Can you work these out from the model? Positions are in its coordinate system, mm. A direction names the side the tool comes from. Give positions to 0.01 mm unless a question says otherwise; leave off trailing zeros. Write each loop counter-clockwise with the first axis right and the second up, starting at its lowest first coordinate (ties: lowest second). Pieces come first, ordered by that corner, then holes. Notation, with made-up numbers: M -11,54.25 L 23,54.25 A18 cw 23,85.25 Z; hole C 19,31 d6. An arc over 180 degrees is marked long. Write each question's results on one line, items separated by ' | '.
from build123d import *

# Parameters (mm, degrees)
SKETCH2_R               = 3
CUT_EXTRUDE1_DEPTH      = 8.5
CUT_EXTRUDE1_DEPTH_BACK = 8.5
DOME1_FACE_RADIUS       = 6
DOME1_HEIGHT            = 2


with BuildPart() as part:
    # Sketch1 → Revolve1 (revolve)
    with BuildSketch(Plane.XY):
        Polygon((57, 0), (0, 0), (0, 6), (18, 6), (18, 5), (20, 5), (20, 7.5), (57, 7.5), align=None)
    revolve(axis=Axis((57, 0, 0), (-1, 0, 0)))

    # Sketch2 → Cut-Extrude1 (cut, two sides)
    with BuildSketch(Plane.XY) as cut_extrude1_sk:
        with Locations((48, 0)):
            Circle(SKETCH2_R)
    extrude(amount=CUT_EXTRUDE1_DEPTH, mode=Mode.SUBTRACT)
    extrude(cut_extrude1_sk.sketch, amount=-CUT_EXTRUDE1_DEPTH_BACK, mode=Mode.SUBTRACT)

    # Dome1: a dome of height H over a round flat face of radius A is a cap of a sphere of radius (A * A + H * H) / (2 * H)
    dome1_r = (DOME1_FACE_RADIUS * DOME1_FACE_RADIUS + DOME1_HEIGHT * DOME1_HEIGHT) / (2 * DOME1_HEIGHT)
    dome1_base = Plane((0, 0, 0), z_dir=(-1, 0, 0))
    with Locations(dome1_base.offset(DOME1_HEIGHT - dome1_r)):
        dome1_ball = Sphere(dome1_r, mode=Mode.PRIVATE)
    add(split(dome1_ball, bisect_by=dome1_base, keep=Keep.TOP, mode=Mode.PRIVATE))


solid = part.part
Item 1: I'm going to push flat-ended pins straight in: pin 1 (6 mm diameter, centred on x = 48.5, y = -3.5, fed in from +Z); pin 2 (1.5 mm diameter, centred on x = 50.5, y = -5, fed in from -Z); pin 3 (3 mm diameter, centred on x = 46, z = -4.5, fed in from +Y); pin 4 (5.5 mm diameter, centred on x = 48, y = 0, fed in from -Z). Where does each tip first touch, or does it pass through?
Geometry says:
pin 1: stops at z = 7.37 | pin 2: stops at z = -6.18 | pin 3: stops at y = 6.87 | pin 4: passes through
Item 2: Thinking about a two-plate mould opening in Y: for faces 1 (the face through (20, -2, 5)), 2 (the face through (45, 0, 0)), 3 (the face through (9, -6, 0)), which applies, +Y half, -Y half, draft (parallel to the pull), parting line (faces both ways), or undercut?
Geometry says:
face 1: draft | face 2: undercut | face 3: parting line
Item 3: For faces 4 (the face through (19.01, -1.08, 4.88)), 5 (the face through (38.759, 7.154, -2.253)), which set-ups out of +Z, -Z, +X, -X, +Y, -Y let a thin tool reach every point of the face, with its end or its side?
Geometry says:
face 4: none | face 5: +X, -X
Item 4: If I drill on line 1 (Y direction, x = 48, z = -4.5); line 2 (Y direction, x = 18.5, z = 0); line 3 (Y direction, x = 48, z = -1.5), over which ranges is the centre line in solid material (lowest first)? Write a range as from..to.
Geometry says:
line 1: y = -6..-3, 3..6 | line 2: y = -5..5 | line 3: y = -7.35..-3, 3..7.35
Item 5: I want a section at B-B, the plane z = 0. Please give me the cut outline in (x, y).
Geometry says:
outline: M 0,-6 L 18,-6 L 18,-5 L 20,-5 L 20,-7.5 L 57,-7.5 L 57,7.5 L 20,7.5 L 20,5 L 18,5 L 18,6 L 0,6 A10 ccw Z; hole C 48,0 d6
Item 6: I want a section at C-C, the plane x = 48. Please give me the cut outline in (y, z).
Geometry says:
outline: M -3,-6.87 L -3,6.87 A7.5 ccw Z; M 3,-6.87 A7.5 ccw 3,6.87 Z
Item 7: I want a section at A-A, the plane y = 0. Please give me the cut outline in (x, z).
Geometry says:
outline: M 0,-6 L 18,-6 L 18,-5 L 20,-5 L 20,-7.5 L 45,-7.5 L 45,7.5 L 20,7.5 L 20,5 L 18,5 L 18,6 L 0,6 A10 ccw Z; M 51,-7.5 L 57,-7.5 L 57,7.5 L 51,7.5 Z
Item 8: I want a section at D-D, the plane x = 25.5. Please give me the cut outline in (y, z), and give its area (3 significant figures).
Geometry says:
outline: C 0,0 d15 | area: 177 mm2
